For this review, take the finished solid that the model builds, in its own axes (mm). Face numbers are marked on the shaded views. A direction names the side the tool comes from. Give positions to 0.01 mm unless a question says otherwise; leave off trailing zeros. Write each loop counter-clockwise with the first axis right and the second up, starting at its lowest first coordinate (ties: lowest second). Pieces come first, ordered by that corner, then holes.
1) Wall thickness on line 1 along X through (y, z) = (17.65, -0.25); line 2 along Y through (x, z) = (1, 1.75); line 3 along Z through (x, y) = (-2, 9.5): over which ranges is each line inside the solid? List them lowest first.
2) Machinability: for the marked faces 4, 5 and 6, which of the approach directions +Z, -Z, +X, -X, +Y, -Y give a long, thin tool a straight path to every point of the face, cutting with its end or side? Answer none if there is none.
3) We need section D-D on y = -3.25. Give the boundary of the cut face in (x, z) (3 decimals).
4) We need section B-B on y = 1.25. Give the boundary of the cut face in (x, z).
5) Draft analysis for pull direction X (two halves, no side actions). For the marked faces 1, 2 and 3, state which applies: pulls with the +X half, pulls with the -X half, needs draft (parallel to the pull), parting line crosses it, or undercut.
6) For P1, Ø0.9, axis at x = -0.5, z = 2, coming from the -Y side; P2, Ø1.2, axis at y = 7.5, z = -5, coming from the +X side; P3, Ø1.5, axis at x = 0.5, y = -1.5, coming from the +Z side (3 decimals), all flat-tipped, find the tip position at first contact; note any pin that passes through.
7) We need section A-A on z = -4.75. Give the boundary of the cut face in (x, y).
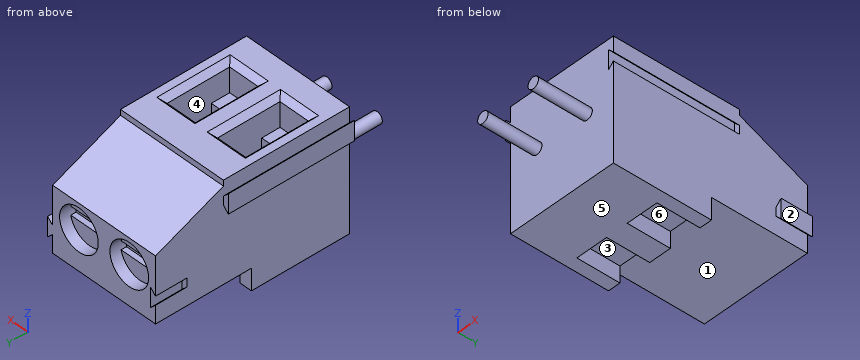
Autodesk Inventor part; units mm, degrees
ref_plane "YZ Plane" through (0, 0, 0) normal (1, 0, 0) x (0, 1, 0)
ref_plane "XZ Plane" through (0, 0, 0) normal (0, 1, 0) x (-1, 0, 0)
ref_plane "XY Plane" through (0, 0, 0) normal (0, 0, 1) x (1, 0, 0)
sketch "Esquisse1" plane through (0, 0, 0) normal (0, 1, 0) x (-1, 0, 0)
  circle A0 centre (0, 0) radius 0.525
  line L0 (2.65, -5.9) -> (-2.65, -5.9)
  line L1 (-2.65, -5.9) -> (-2.65, 5.3)
  line L2 (-2.65, 5.3) -> (2.65, 5.3)
  line L3 (2.65, 5.3) -> (2.65, -5.9)
  point P0 (0, 5.3)
  dimension "d0" = 1.05
  dimension "d1" = 11.2
  dimension "d2" = 5.3
  dimension "d4" = 2.65
extrude "Extrusion1" add sketch "Esquisse1" along normal blind 18 contours A0 | L0 L1 L2 L3
sketch "Esquisse8" plane through (0, 0, 0) normal (0, 1, 0) x (-1, 0, 0)
  line L0 (-7.73, 3.1) -> (-7.23, 2.6)
  line L1 (-7.23, 2.6) -> (-7.23, 4.4)
  line L2 (-7.23, 4.4) -> (-7.73, 3.9)
  line L3 (-7.73, 3.9) -> (-7.73, 3.1)
  line L4 (2.65, 3.1) -> (3.15, 2.6)
  line L5 (3.15, 2.6) -> (3.15, 4.4)
  line L6 (3.15, 4.4) -> (2.65, 3.9)
  line L7 (2.65, 3.9) -> (2.65, 3.1)
  line L8 (-8.23, -0.95) -> (-8.23, -2.75)
  line L9 (-8.23, -2.75) -> (-7.73, -2.25)
  line L10 (-7.73, -2.25) -> (-7.73, -1.45)
  line L11 (-7.73, -1.45) -> (-8.23, -0.95)
  line L12 (2.15, -0.95) -> (2.15, -2.75)
  line L13 (2.15, -2.75) -> (2.65, -2.25)
  line L14 (2.65, -2.25) -> (2.65, -1.45)
  line L15 (2.65, -1.45) -> (2.15, -0.95)
  line L16 (0, 0) -> (0, -11.21) construction
  dimension "d45" = 45
  dimension "d46" = 0.8
  dimension "d47" = 1.8
  dimension "d48" = 4.4
  dimension "d49" = 45
  dimension "d50" = 0.8
  dimension "d51" = 1.8
  dimension "d53" = 7.73
  dimension "d56" = 2.65
  dimension "d105" = 1.8
  dimension "d106" = 45
  dimension "d107" = 0.8
  dimension "d108" = 135
  dimension "d109" = 1.8
  dimension "d110" = 45
  dimension "d111" = 0.8
  dimension "d112" = 135
  dimension "d119" = 2.75
sketch "Esquisse9" plane through (0, 18, 0) normal (0, 1, 0) x (1, 0, 0)
  line L0 (-2.15, 2.75) -> (-2.65, 2.25)
  line L1 (-2.65, 2.25) -> (-2.65, 1.45)
  line L2 (-2.15, 0.95) -> (-2.15, 2.75)
  line L3 (-2.65, 1.45) -> (-2.15, 0.95)
  line L4 (8.23, 2.75) -> (7.73, 2.25)
  line L5 (8.23, 0.95) -> (8.23, 2.75)
  line L6 (7.73, 1.45) -> (8.23, 0.95)
  line L7 (7.73, 2.25) -> (7.73, 1.45)
sketch "Esquisse2" plane through (2.65, 0, 5.3) normal (1, 0, 0) x (0, 0, -1)
  line L0 (11.2, 0) -> (0, 0)
  line L1 (11.2, 0) -> (11.2, 18) construction
  line L2 (0, 18) -> (11.2, 18) construction
  line L3 (0, 0) -> (0, 18) construction
  line L4 (3.2, 18) -> (9.2, 18)
  line L5 (9.2, 18) -> (9.2, 9.1)
  line L6 (9.2, 9.1) -> (11.2, 9.1)
  line L7 (0, 11.7) -> (0.52, 11.7)
  line L8 (0.52, 11.7) -> (3.2, 18)
  line L9 (0, 11.7) -> (0, 18)
  line L10 (0, 18) -> (3.2, 18)
  line L11 (9.2, 18) -> (11.2, 18)
  line L12 (11.2, 18) -> (11.2, 9.1)
  point P0 (5.3, 0)
  dimension "d7" = 0.52
  dimension "d8" = 6
  dimension "d9" = 9.1
  dimension "d10" = 2
  dimension "d11" = 11.7
extrude "Extrusion2" cut sketch "Esquisse2" against normal through all
sketch "Esquisse3" plane through (0, 18, 0) normal (0, 1, 0) x (1, 0, 0)
  line L0 (-2.65, -2.1) -> (2.65, -2.1)
  line L1 (2.65, -2.1) -> (2.65, 3.9)
  line L2 (2.65, 3.9) -> (-2.65, 3.9)
  line L3 (-2.65, 3.9) -> (-2.65, -2.1)
  circle A0 centre (0, 0.25) radius 1.95
  point P0 (0, 0)
  point P1 (0, -2.1)
  dimension "d14" = 3.9
  dimension "d15" = 1.7
extrude "Extrusion3" cut sketch "Esquisse3" against normal blind 1 contours A0
sketch "Esquisse4" plane through (0, 17, -0.25) normal (0, 1, 0) x (1, 0, 0)
  circle A0 centre (0, 0) radius 1.95
  line L0 (-1.9085, 0.4) -> (1.9085, 0.4)
  line L1 (-1.9085, -0.4) -> (1.9085, -0.4)
  point P0 (0, -0.25)
  dimension "d18" = 0.8
extrude "Extrusion4" cut sketch "Esquisse4" against normal blind 0.5 contours A0 L1 L0
sketch "Esquisse5" plane through (-2.65, 0, 5.3) normal (0, 0, 1) x (1, 0, 0)
  line L0 (5.3, 11.7) -> (0, 11.7)
  line L1 (0, 0) -> (0, 11.7)
  line L2 (5.3, 0) -> (0, 0)
  line L3 (5.3, 0) -> (5.3, 11.7)
  line L4 (1.225, 8.5) -> (4.075, 8.5)
  line L5 (4.075, 8.5) -> (4.075, 2.7)
  line L6 (4.075, 2.7) -> (1.225, 2.7)
  line L7 (1.225, 2.7) -> (1.225, 8.5)
  point P0 (2.65, 0)
  dimension "d21" = 1.225
  dimension "d22" = 2.85
  dimension "d23" = 5.8
  dimension "d24" = 2.7
  dimension "d25" = 1.225
extrude "Extrusion5" cut sketch "Esquisse5" against normal blind 2.77 contours L4 L5 L6 L7
chamfer "Chanfrein1" distance 0.5 angle 45 4 edges at (-1.425, 5.6, 5.3) (0, 8.5, 5.3) (1.425, 5.6, 5.3) (0, 2.7, 5.3)
sketch "Esquisse6" plane through (-2.65, 0, 2.53) normal (0, 0, 1) x (1, 0, 0)
  line L0 (1.225, 8.5) -> (4.075, 8.5)
  line L1 (1.225, 2.7) -> (1.225, 8.5)
  line L2 (4.075, 2.7) -> (1.225, 2.7)
  line L3 (4.075, 8.5) -> (4.075, 2.7)
  line L4 (1.225, 4.4) -> (4.075, 4.4)
  point P0 (2.65, 0)
  dimension "d31" = 1.7
extrude "Extrusion6" cut sketch "Esquisse6" against normal blind 3 contours L0 L3 L4 L1
sketch "Esquisse7" plane through (2.65, 0, -5.9) normal (0, 0, -1) x (-1, 0, 0)
  line L0 (5.3, 9.1) -> (0, 9.1) construction
  line L1 (0, 0) -> (0, 9.1) construction
  line L2 (5.3, 0) -> (0, 0) construction
  line L3 (5.3, 0) -> (5.3, 9.1) construction
  line L4 (1.15, 9.1) -> (1.15, 5.1)
  line L5 (1.15, 5.1) -> (4.15, 5.1)
  line L6 (4.15, 5.1) -> (4.15, 9.1)
  line L7 (4.15, 9.1) -> (1.15, 9.1)
  point P0 (2.65, 0)
  dimension "d34" = 3
  dimension "d35" = 4
  dimension "d36" = 1.15
  dimension "d37" = 1.15
extrude "Extrusion7" cut sketch "Esquisse7" against normal blind 1.5
extrude "Extrusion8" add sketch "Esquisse1" against normal blind 5 contours A0
sketch "SilkS" plane through (0, 18, 0) normal (0, 1, 0) x (1, 0, 0)
  line L0 (2.65, -5.3) -> (-10.27, -5.3)
  line L1 (-10.27, 5.9) -> (2.65, 5.9)
  line L2 (-10.27, 5.9) -> (-10.27, -5.3)
  line L3 (2.65, 5.9) -> (2.65, -5.3)
  point P0 (0, 0)
  dimension "d121" = 10.27
sketch "CrtYd" plane through (0, 18, 0) normal (0, 1, 0) x (1, 0, 0)
  line L0 (7.73, -3.1) -> (7.23, -2.6)
  line L1 (7.23, -2.6) -> (7.23, -4.4)
  line L2 (7.73, -3.9) -> (7.73, -3.1)
  line L3 (7.23, -4.4) -> (7.73, -3.9)
  line L4 (-2.65, -3.1) -> (-3.15, -2.6)
  line L5 (-3.15, -2.6) -> (-3.15, -4.4)
  line L6 (-2.65, -3.9) -> (-2.65, -3.1)
  line L7 (-3.15, -4.4) -> (-2.65, -3.9)
  line L8 (2.65, 2.35) -> (2.65, 1.55)
  line L9 (3.15, 2.85) -> (2.65, 2.35)
  line L10 (3.15, 1.05) -> (3.15, 2.85)
  line L11 (2.65, 1.55) -> (3.15, 1.05)
  line L12 (-2.15, 2.85) -> (-2.65, 2.35)
  line L13 (-2.15, 1.05) -> (-2.15, 2.85)
  line L14 (-2.65, 2.35) -> (-2.65, 1.55)
  line L15 (-2.65, 1.55) -> (-2.15, 1.05)
  circle A0 centre (0, 0.25) radius 1.95 construction
  line L16 (1.425, -4.8) -> (-1.425, -4.8) construction
  line L17 (-1.925, -5.3) -> (-1.425, -4.8) construction
  line L18 (-1.925, -5.3) -> (1.925, -5.3) construction
  line L19 (1.925, -5.3) -> (1.425, -4.8) construction
  line L20 (1.425, -4.8) -> (-1.425, -4.8) construction
  line L21 (1.425, -4.8) -> (1.425, -2.53) construction
  line L22 (1.425, -2.53) -> (-1.425, -2.53) construction
  line L23 (-1.425, -4.8) -> (-1.425, -2.53) construction
  circle A1 centre (0, 0.25) radius 1.95
  line L24 (1.425, -2.53) -> (1.425, -4.8)
  line L25 (1.425, -4.8) -> (1.925, -5.3)
  line L26 (1.925, -5.3) -> (-1.925, -5.3)
  line L27 (-1.925, -5.3) -> (-1.425, -4.8)
  line L28 (-1.425, -4.8) -> (-1.425, -2.53)
  line L29 (-1.425, -2.53) -> (1.425, -2.53)
  line L30 (1.425, -4.8) -> (-1.425, -4.8)
  circle A2 centre (5.08, 0.25) radius 1.95
  line L31 (3.655, -2.53) -> (6.505, -2.53)
  line L32 (3.655, -4.8) -> (3.655, -2.53)
  line L33 (6.505, -2.53) -> (6.505, -4.8)
  line L34 (6.505, -4.8) -> (3.655, -4.8)
  line L35 (7.005, -5.3) -> (3.155, -5.3)
  line L36 (6.505, -4.8) -> (7.005, -5.3)
  line L37 (3.155, -5.3) -> (3.655, -4.8)
  line L38 (-2.65, -3.9) -> (-2.65, -5.3)
  line L39 (-2.65, -5.3) -> (7.73, -5.3)
  line L40 (7.73, -5.3) -> (7.73, -3.9)
  line L41 (2.65, -3.1) -> (2.65, 1.55)
  line L42 (2.65, 2.35) -> (2.65, 5.9)
  line L43 (2.65, 5.9) -> (-2.65, 5.9)
  line L44 (-2.65, 5.9) -> (-2.65, 2.35)
  line L45 (-2.65, 1.55) -> (-2.65, -3.1)
  point P0 (0, 0)
  dimension "d98" = 5.08
pattern_linear "Réseau rectangulaire1" count 2 spacing 5.08 along (1, 0, 0)
extrude "Extrusion9" cut sketch "Esquisse8" along normal up to surface (11.7 mm away) contours L3 L2 L1 L0
extrude "Extrusion10" add sketch "Esquisse8" along normal up to surface (11.7 mm away) contours L7 L6 L5 L4
extrude "Extrusion11" add sketch "Esquisse9" against normal blind 2.9 contours L5 L6 L7 L4
extrude "Extrusion12" cut sketch "Esquisse9" against normal blind 2.9 contours L2 L3 L1 L0
equation "\"d21\" = d25"
equation "\"d36\" = d37"
properties part number "bornier_vert_5.08_variable"
Results list:
1. line 1: x = -2.65 to -1.95, 1.95 to 3.13, 7.03 to 7.73
1. line 2: y = 0 to 4.4, 8.5 to 18
1. line 3: z = -3.9 to 5.3
2. face 4: +Z
2. face 5: -Z, +X, -X, +Y, -Y
2. face 6: -Z, +Y
3. outline: circle Ø1.05 at (0, 0); circle Ø1.05 at (5.08, 0)
4. outline: (-3.15, 2.6) - (-2.65, 3.1) - (-2.65, -5.9) - (7.73, -5.9) - (7.73, 3.1) - (7.23, 2.6) - (7.23, 4.4) - (7.73, 3.9) - (7.73, 5.3) - (-2.65, 5.3) - (-2.65, 3.9) - (-3.15, 4.4) - close
5. face 1: needs draft
5. face 2: pulls with the +X half
5. face 3: undercut
6. P1: stops at y = 0
6. P2: stops at x = 7.73
6. P3: stops at z = 0.525
7. outline: (-2.65, 0) - (7.73, 0) - (7.73, 9.1) - (6.58, 9.1) - (6.58, 5.1) - (3.58, 5.1) - (3.58, 9.1) - (1.5, 9.1) - (1.5, 5.1) - (-1.5, 5.1) - (-1.5, 9.1) - (-2.65, 9.1) - close
